Autodesk Inventor part; units mm, degrees
ref_plane "YZ Plane" through (0, 0, 0) normal (1, 0, 0) x (0, 1, 0)
ref_plane "XZ Plane" through (0, 0, 0) normal (0, 1, 0) x (-1, 0, 0)
ref_plane "XY Plane" through (0, 0, 0) normal (0, 0, 1) x (1, 0, 0)
sketch "Sketch1" plane through (0, 0, 0) normal (0, 0, 1) x (1, 0, 0)
  circle A0 centre (13.4234, -7.75) radius 1.5
  circle A1 centre (-13.4234, -7.75) radius 1.5
  circle A2 centre (0, 15.5) radius 1.5
  circle A3 centre (-13.4234, 7.75) radius 1.5
  circle A4 centre (0, -15.5) radius 1.5
  circle A5 centre (13.4234, 7.75) radius 1.5
  circle A6 centre (7, 0) radius 7
  circle A7 centre (0, 0) radius 18.5
  circle A8 centre (7, 0) radius 7.5
  line L0 (16.9115, 7.5) -> (51.9115, 7.5)
  line L1 (51.9115, 7.5) -> (51.9115, -7.5)
  line L2 (51.9115, -7.5) -> (16.9115, -7.5)
  line L3 (51.9115, -10) -> (58.9115, -10)
  line L4 (58.9115, -10) -> (58.9115, 10)
  line L5 (58.9115, 10) -> (51.9115, 10)
  line L6 (51.9115, 10) -> (51.9115, -10)
  point P0 (0, 0)
  point P1 (51.9115, -7.5)
  dimension "d0" = 15
  dimension "d1" = 35
  dimension "d2" = 20
  dimension "d3" = 7
  dimension "d4" = 2.5
  dimension "d5" = 0
extrude "Extrusion1" add sketch "Sketch1" along normal blind 8 contours A7 | A7 L0 L1 L2 | L6 L5 L4 L3 L1
sketch "Sketch2" plane through (58.9115, -10, 0) normal (1, 0, 0) x (0, 0, -1)
  line L0 (-23, 20) -> (15, 20)
  line L1 (15, 20) -> (15, 0)
  line L2 (15, 0) -> (-23, 0)
  line L3 (-23, 0) -> (-23, 20)
  line L4 (0, 20) -> (-8, 20)
  line L5 (-8, 0) -> (-8, 20)
  circle A0 centre (7.5, 10) radius 2.25
  circle A1 centre (-15.5, 10) radius 2.25
  point P0 (0, 10)
  dimension "d8" = 20
  dimension "d9" = 0
  dimension "d10" = 38
  dimension "d11" = 15
  dimension "d12" = 4.5
  dimension "d13" = 4.5
  dimension "d14" = 7.5
  dimension "d15" = 7.5
extrude "Extrusion2" add sketch "Sketch2" against normal blind 8
fillet "Fillet1" radius 20 2 edges at (16.9115, 7.5, 4) (16.9115, -7.5, 4)
equation "\"d14\" = d15"
properties part number "DCMotorHolder"
Source: CAD feature listing. Evaluate the final solid. Frame: model axes, mm. A direction names the side the tool comes from. Give positions to 0.01 mm unless a question says otherwise; leave off trailing zeros. Write each loop counter-clockwise with the first axis right and the second up, starting at its lowest first coordinate (ties: lowest second). Pieces come first, ordered by that corner, then holes. Notation, with made-up numbers: M 81,-33.75 L 92,-33.75 A31 cw 92,2.25 Z; hole C -23.75,49 d11. An arc over 180 degrees is marked long. Answer as a JSON object with one key per item and string values.
Q1. Access query for faces 5 (the face through (16, 0, 0)), 6 (the face through (55, 10, 4)), 7 (the face through (16, 0, 8)), 8 (the face through (39, -7.5, 4)). Directions: +Z, -Z, +X, -X, +Y, -Y. A direction counts if a zero-diameter tool reaches every point of the face in a straight line with its end or side. Return the directions, or none.
Geometry check:
{"face 5": "-Z, -X, +Y, -Y", "face 6": "+Z, -Z, +X, +Y", "face 7": "+Z, -X, +Y, -Y", "face 8": "+Z, -Z, -Y"}
Q2. Mould query, pull axis X, two halves, no side actions, for faces 1 (the face through (58.912, 0, 4)), 2 (the face through (55, -10, 4)), 3 (the face through (19.285, 9.025, 4.056)), 4 (the face through (39, 7.5, 4)). Classes: +X half, -X half, draft (parallel to the pull), parting line (faces both ways), or undercut.
Geometry check:
{"face 1": "+X half", "face 2": "draft", "face 3": "undercut", "face 4": "undercut"}
Q3. Cut plane D-D, the plane y = -5. Return the cut outline in (x, z).
Geometry check:
{"outline": "M -17.81,0 L 1.41,0 L 1.41,8 L -17.81,8 Z; M 12.59,0 L 50.91,0 L 50.91,-15 L 58.91,-15 L 58.91,23 L 50.91,23 L 50.91,8 L 12.59,8 Z"}
Q4. Ray query, line 1 along Z through (x, y) = (-10.5, -13); line 2 along Y through (x, z) = (53.75, 15.5); line 3 along X through (y, z) = (-2.5, 18). Return the intervals inside material, ascending.
Geometry check:
{"line 1": "z = 0 to 8", "line 2": "y = -10 to -2.25, 2.25 to 10", "line 3": "x = 50.91 to 58.91"}
Q5. Contact query for flat-ended pins moving along their axis: P1, Ø5, axis at x = 13.42, y = 7.75, coming from the +Z side; P2, Ø6, axis at y = 11, z = 7, coming from the -X side; P3, Ø4, axis at x = 54.5, z = 5, coming from the -Y side. Output: stop coordinate, or through.
Geometry check:
{"P1": "stops at z = 8", "P2": "stops at x = -16.68", "P3": "stops at y = -10"}
Q6. Cut plane B-B, the plane y = 1. Return the cut outline in (x, z), then the cut area to 3 significant figures.
Geometry check:
{"outline": "M -18.47,0 L -0.43,0 L -0.43,8 L -18.47,8 Z; M 14.43,0 L 50.91,0 L 50.91,-5.48 L 58.91,-5.48 L 58.91,13.48 L 50.91,13.48 L 50.91,8 L 14.43,8 Z; M 50.91,-15 L 58.91,-15 L 58.91,-9.52 L 50.91,-9.52 Z; M 50.91,17.52 L 58.91,17.52 L 58.91,23 L 50.91,23 Z", "area": "676 mm^2"}
Q7. Cut plane A-A, the plane z = -7.5. Return the cut outline in (x, y).
Geometry check:
{"outline": "M 50.91,-10 L 58.91,-10 L 58.91,-2.25 L 50.91,-2.25 Z; M 50.91,2.25 L 58.91,2.25 L 58.91,10 L 50.91,10 Z"}
Q8. Cut plane C-C, the plane x = 7. Return the cut outline in (y, z), then the cut area to 3 significant figures.
Geometry check:
{"outline": "M -17.12,0 L -7.5,0 L -7.5,8 L -17.12,8 Z; M 7.5,0 L 17.12,0 L 17.12,8 L 7.5,8 Z", "area": "154 mm^2"}
